Input: part model. Units: mm. Frame: model coordinates. Face numbers are marked on the shaded views. A direction names the side the tool comes from. Give positions to 0.01 mm unless a question says otherwise; leave off trailing zeros. Loops run counter-clockwise (first coordinate to the right, second up) from the corner with the lowest first, then second, coordinate; pieces in that order, holes last.
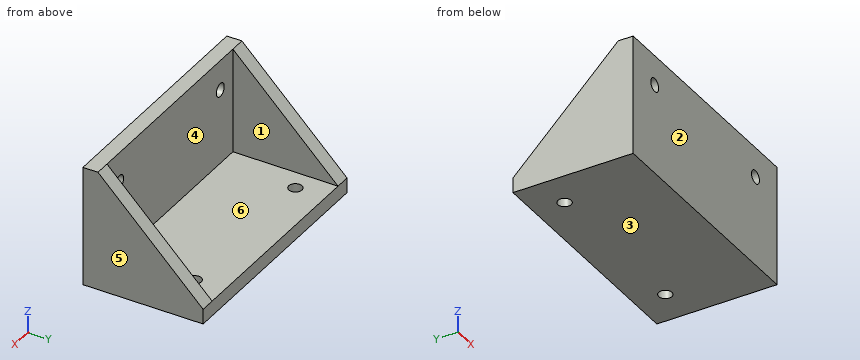
from build123d import *

# Parameters (mm, degrees)
SKETCH1_W           = 80
SKETCH1_H           = 40
BOSS_EXTRUDE1_DEPTH = 5
SKETCH2_W           = 80
SKETCH2_H           = 5
BOSS_EXTRUDE2_DEPTH = 35
BOSS_EXTRUDE3_DEPTH = 5
BOSS_EXTRUDE4_DEPTH = 5
SKETCH5_R           = 2.2
CUT_EXTRUDE1_DEPTH  = 6
SKETCH6_R           = 2.2
CUT_EXTRUDE2_DEPTH  = 6


with BuildPart() as part:
    # Sketch1 → Boss-Extrude1 (new body)
    with BuildSketch(Plane(origin=(0, 0, 0), x_dir=(1, 0, 0), z_dir=(0, 1, 0))):
        Rectangle(SKETCH1_W, SKETCH1_H)
    extrude(amount=BOSS_EXTRUDE1_DEPTH)

    # Sketch2 → Boss-Extrude2 (add)
    with BuildSketch(Plane(origin=(0, 5, 0), x_dir=(1, 0, 0), z_dir=(0, 1, 0))):
        with Locations((0, 17.5)):
            Rectangle(SKETCH2_W, SKETCH2_H)
    extrude(amount=BOSS_EXTRUDE2_DEPTH)

    # Sketch3 → Boss-Extrude3 (add)
    with BuildSketch(Plane.ZY.offset(40)):
        Polygon((-15, 40), (20, 5), (-15, 5), align=None)
    extrude(amount=-BOSS_EXTRUDE3_DEPTH)

    # Sketch4 → Boss-Extrude4 (add)
    with BuildSketch(Plane(origin=(40, 0, 0), x_dir=(0, 0, -1), z_dir=(1, 0, 0))):
        Polygon((15, 40), (-20, 5), (15, 5), align=None)
    extrude(amount=-BOSS_EXTRUDE4_DEPTH)

    # Sketch5 → Cut-Extrude1 (cut, through all)
    with BuildSketch(Plane(origin=(0, 5, 0), x_dir=(1, 0, 0), z_dir=(0, 1, 0))):
        with Locations((-28, -10)):
            Circle(SKETCH5_R)
        with Locations((28, -10)):
            Circle(SKETCH5_R)
    extrude(amount=-CUT_EXTRUDE1_DEPTH, mode=Mode.SUBTRACT)

    # Sketch6 → Cut-Extrude2 (cut, through all)
    with BuildSketch(Plane.XY.offset(-15)):
        with Locations((-28, 30)):
            Circle(SKETCH6_R)
        with Locations((28, 30)):
            Circle(SKETCH6_R)
    extrude(amount=-CUT_EXTRUDE2_DEPTH, mode=Mode.SUBTRACT)


solid = part.part
(1) Mould query, pull axis X, two halves, no side actions, for the marked faces 3, 4, 5 and 6. Classes: +X half, -X half, draft (parallel to the pull), parting line (faces both ways), or undercut.
Values follow:
face 3: draft
face 4: undercut
face 5: +X half
face 6: undercut
(2) Cut plane C-C (y = 30). Return the cut outline in (x, z), and give its area (3 significant figures).
Values follow:
outline: (-40, -20) - (-30.2, -20) - (-30.2, -15) - (-35, -15) - (-35, -5) - (-40, -5) - close; (-25.8, -20) - (25.8, -20) - (25.8, -15) - (-25.8, -15) - close; (30.2, -20) - (40, -20) - (40, -5) - (35, -5) - (35, -15) - (30.2, -15) - close
area: 456 mm2
(3) Ray query, probe 1 along Y at (x, z) = (28, -18); probe 2 along X at (y, z) = (24, -1); probe 3 along X at (y, z) = (2, 10). Return the intervals inside material, ascending.
Values follow:
probe 1: y = 0 to 27.8, 32.2 to 40
probe 2: x = -40 to -35, 35 to 40
probe 3: x = -40 to -30.2, -25.8 to 25.8, 30.2 to 40
(4) Cut plane B-B (z = 10). Return the cut outline in (x, y).
Values follow:
outline: (-40, 0) - (-30.2, 0) - (-30.2, 5) - (-35, 5) - (-35, 15) - (-40, 15) - close; (-25.8, 0) - (25.8, 0) - (25.8, 5) - (-25.8, 5) - close; (30.2, 0) - (40, 0) - (40, 15) - (35, 15) - (35, 5) - (30.2, 5) - close
(5) Cut plane D-D (y = 23). Return the cut outline in (x, z), and give its area (3 significant figures).
Values follow:
outline: (-40, -20) - (40, -20) - (40, 2) - (35, 2) - (35, -15) - (-35, -15) - (-35, 2) - (-40, 2) - close
area: 570 mm2
(6) Pin query (flat end, axial travel): pin 1 Ø7 at (x, z) = (28, 10) entering from +Y; pin 2 Ø17.5 at (x, y) = (11.5, 30.5) entering from +Z. Return the tip coordinate at first contact, or that it passes through.
Values follow:
pin 1: stops at y = 5
pin 2: stops at z = -15
(7) Cut plane A-A (x = -28). Return the cut outline in (y, z).
Values follow:
outline: (0, -20) - (27.8, -20) - (27.8, -15) - (5, -15) - (5, 7.8) - (0, 7.8) - close; (0, 12.2) - (5, 12.2) - (5, 20) - (0, 20) - close; (32.2, -20) - (40, -20) - (40, -15) - (32.2, -15) - close
(8) Reachability of the marked faces 1 and 2 from +Z, -Z, +X, -X, +Y, -Y: full face, straight path, thin tool, end or side. Return the list, or none.
Values follow:
face 1: +Z, +Y
face 2: +Z, -Z, +X, -X, -Y
